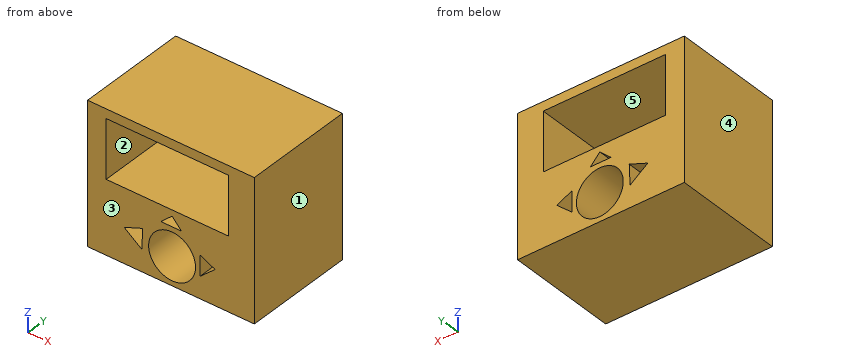
```python
from build123d import *

# Parameters (mm, degrees)
F0_R     = 16.183835
F1_DEPTH = 76.2


with BuildPart() as f1:
    # F0 (on Front) → F1 (new body)
    with BuildSketch(Plane.XZ):
        Polygon((56.764722, 57.920564), (0, 57.920564), (-58.305845, 57.920564), (-58.305845, -39.170228), (56.764722, -39.170228), align=None)
        Polygon((-33.118952, -15.107391), (-20.291461, -10.14573), (-20.851416, -24.272695), align=None, mode=Mode.SUBTRACT)
        with Locations((0, -19.649327)):
            Circle(F0_R, mode=Mode.SUBTRACT)
        Polygon((19.264044, -24.272695), (19.264044, -10.14573), (29.703761, -15.107391), align=None, mode=Mode.SUBTRACT)
        Polygon((6.474859, 0), (-7.705619, 0), (0, 7.063483), align=None, mode=Mode.SUBTRACT)
        Polygon((-2.311687, 51.499214), (0, 51.499214), (39.041799, 51.499214), (39.041799, 11.173147), (-45.463149, 11.173147), (-45.463149, 51.499214), align=None, mode=Mode.SUBTRACT)
    extrude(amount=F1_DEPTH)


solid = f1.part
```
Work out the finished part from the listing and answer in its coordinate system (mm). Face numbers are marked on the shaded views. A direction names the side the tool comes from. Coordinates: 2 decimals unless noted, no trailing zeros. Loops run counter-clockwise (first coordinate to the right, second up) from the corner with the lowest first, then second, coordinate; pieces in that order, holes last. Notation, with made-up numbers: M 79,65.25 L 110,65.25 A18 cw 110,80.25 Z; hole C -4.5,87 d7. An arc over 180 degrees is marked long. Use CSV: the item, a comma, the result in double quotes. Start each with the question number.
(1) Find section B-B, the plane x = 13. Give the vertices of the cut face in (y, z).
(2) Consider line 1 (Z direction, x = 0, y = -22); line 2 (Z direction, x = 35, y = -71.5); line 3 (X direction, y = -37, z = 21). Determine where each line is inside the solid, lowest interval first.
(3) Find section D-D, the plane z = -12. Give the vertices of the cut face in (x, y).
(4) Find section C-C, the plane y = -14.5. Give the vertices of the cut face in (x, z).
(5) For a pull along X with two mould halves and no side action, classify the marked faces 1, 2 and 3 as +X half, -X half, draft (parallel to the pull), parting line (faces both ways), or undercut.
(6) Find section A-A, the plane z = -29. Give the vertices of the cut face in (x, y), then the cut area to 3 significant figures.
(7) Given pin 1 Ø3 at (x, z) = (9, -9.5) entering from +Y, flat-ended and moving along its own axis, determine where the tip first touches the part or whether it passes through.
(8) For the marked faces 4 and 5, determine the directions among +Z, -Z, +X, -X, +Y, -Y from which every point of the face is accessible in a straight line to the end or side of a thin tool.
Recorded:
1,outline,"M -76.2,-39.17 L 0,-39.17 L 0,-29.29 L -76.2,-29.29 Z; M -76.2,-10.01 L 0,-10.01 L 0,11.17 L -76.2,11.17 Z; M -76.2,51.5 L 0,51.5 L 0,57.92 L -76.2,57.92 Z"
2,line 1,"z = -39.17 to -35.83, -3.47 to 0, 7.06 to 11.17, 51.5 to 57.92"
2,line 2,"z = -39.17 to 11.17, 51.5 to 57.92"
2,line 3,"x = -58.31 to -45.46, 39.04 to 56.76"
3,outline,"M -58.31,-76.2 L -25.09,-76.2 L -25.09,0 L -58.31,0 Z; M -20.36,-76.2 L -14.26,-76.2 L -14.26,0 L -20.36,0 Z; M 14.26,-76.2 L 19.26,-76.2 L 19.26,0 L 14.26,0 Z; M 23.17,-76.2 L 56.76,-76.2 L 56.76,0 L 23.17,0 Z"
4,outline,"M -58.31,-39.17 L 56.76,-39.17 L 56.76,57.92 L -58.31,57.92 Z; hole M -45.46,11.17 L 39.04,11.17 L 39.04,51.5 L -45.46,51.5 Z; hole M -33.12,-15.11 L -20.85,-24.27 L -20.29,-10.15 Z; hole C 0,-19.65 d32.37; hole M -7.71,0 L 6.47,0 L 0,7.06 Z; hole M 19.26,-24.27 L 29.7,-15.11 L 19.26,-10.15 Z"
5,face 1,"+X half"
5,face 2,"undercut"
5,face 3,"draft"
6,outline,"M -58.31,-76.2 L -13.21,-76.2 L -13.21,0 L -58.31,0 Z; M 13.21,-76.2 L 56.76,-76.2 L 56.76,0 L 13.21,0 Z"
6,area,"6,760 mm^2"
7,pin 1,"passes through"
8,face 4,"+Z, -Z, -X, +Y, -Y"
8,face 5,"+Y, -Y"
